The listing builds one solid part. Answer for the finished solid, in the listing's coordinates (mm). A direction names the side the tool comes from. Give positions to 0.01 mm unless a question says otherwise; leave off trailing zeros. Write each loop counter-clockwise with the first axis right and the second up, starting at its lowest first coordinate (ties: lowest second). Pieces come first, ordered by that corner, then holes. Notation, with made-up numbers: M -30,23.25 L -1,23.25 A32 cw -1,59.25 Z; hole C -38,-2.5 d4. An arc over 180 degrees is marked long. Return JSON: item names as keys, results as strings.
from build123d import *

# Parameters (mm, degrees)
F0_W     = 228.6
F0_H     = 182.245
F1_DEPTH = 7.62
F2_W     = 228.6
F2_H     = 158.7754
F3_DEPTH = 6.731
F4_W     = 2.54
F4_H     = 2.54
F5_DEPTH = 228.6
F6_W     = 20.32
F6_H     = 20.32
F7_DEPTH = 76.2
F8_W     = 81.5747073555
F8_H     = 20.3200148768
F9_DEPTH = 19.05
F10_R    = 10.16


with BuildPart() as f1:
    # F0 (on Top) → F1 (new body)
    with BuildSketch(Plane.XY):
        with Locations((53.7457112223, 38.7887536495)):
            Rectangle(F0_W, F0_H)
    extrude(amount=F1_DEPTH)

    # F2 (on face) → F3 (join)
    with BuildSketch(Plane(origin=(0, 0, 0), x_dir=(1, 0, 0), z_dir=(0, 0, -1))):
        with Locations((53.7457112223, -38.7887536495)):
            Rectangle(F2_W, F2_H)
    extrude(amount=F3_DEPTH)

    # F4 (on face) → F5 (join)
    with BuildSketch(Plane.YZ.offset(168.0457112223)):
        with Locations((119.4464536495, -5.461)):
            Rectangle(F4_W, F4_H)
        with Locations((-41.8689463505, -5.461)):
            Rectangle(F4_W, F4_H)
    extrude(amount=-F5_DEPTH)

    # F6 (on face) → F7 (join)
    with BuildSketch(Plane.XY.offset(7.62)):
        with Locations((0, 38.7887536495)):
            Rectangle(F6_W, F6_H)
        Polygon((101.8946701026, 48.9487536495), (91.7346701026, 48.9487536495), (91.7346701026, 28.6287536495), (112.0546701026, 28.6287536495), (112.0546701026, 48.9487536495), align=None)
    extrude(amount=F7_DEPTH)

    # F8 (on face) → F9 (join)
    with BuildSketch(Plane.XY.offset(83.82)):
        with Locations((50.9473536777, 38.7887610879)):
            Rectangle(F8_W, F8_H)
    extrude(amount=-F9_DEPTH)

    # F10
    f10_edges = [f1.edges().sort_by_distance(p)[0] for p in [
        (-10.16, 38.788754, 83.82),
        (112.05467, 38.788754, 83.82),
        (10.16, 38.788754, 64.77),
        (91.73467, 38.788754, 64.77),
    ]]
    fillet(f10_edges, radius=F10_R)


solid = f1.part
Item 1: Which of the six approach directions +Z, -Z, +X, -X, +Y, -Y give full straight-line access (tool end or side, diameter ignored) to faces 1 (the flat face through (-10.16, 39, 40)), 2 (the flat face through (50, 39, 64.77)), 3 (the flat face through (52, 124, 0)), 4 (the flat face through (50, 28.629, 72))?
Geometry results:
{"face 1": "+Z, -X, +Y, -Y", "face 2": "+Y, -Y", "face 3": "+X, -X, +Y", "face 4": "+Z, +X, -X, -Y"}
Item 2: A cutting plane is placed at D-D, the plane y = 75.5. Write down the section's boundary in (x, z), plus the area to 3 significant figures.
Geometry results:
{"outline": "M -60.55,-6.73 L 168.05,-6.73 L 168.05,7.62 L -60.55,7.62 Z", "area": "3,280 mm2"}
Item 3: A cutting plane is placed at A-A, the plane x = 62. Write down the section's boundary in (y, z).
Geometry results:
{"outline": "M -52.33,0 L -40.6,0 L -40.6,-4.19 L -43.14,-4.19 L -43.14,-6.73 L 120.72,-6.73 L 120.72,-4.19 L 118.18,-4.19 L 118.18,0 L 129.91,0 L 129.91,7.62 L -52.33,7.62 Z; M 28.63,64.77 L 48.95,64.77 L 48.95,83.82 L 28.63,83.82 Z"}
Item 4: A cutting plane is placed at C-C, the plane x = -45. Write down the section's boundary in (y, z), plus the area to 3 significant figures.
Geometry results:
{"outline": "M -52.33,0 L -40.6,0 L -40.6,-4.19 L -43.14,-4.19 L -43.14,-6.73 L 120.72,-6.73 L 120.72,-4.19 L 118.18,-4.19 L 118.18,0 L 129.91,0 L 129.91,7.62 L -52.33,7.62 Z", "area": "2,470 mm2"}
Item 5: Determine the mould class of faces 5 (the cylindrical face through (88.68, 38.65, 61.87)), 6 (the flat face through (52, -46, 0)), 7 (the flat face through (112.055, 39, 40)) for opening direction X: +X half, -X half, draft (parallel to the pull), parting line (faces both ways), or undercut.
Geometry results:
{"face 5": "undercut", "face 6": "draft", "face 7": "+X half"}
Item 6: A cutting plane is placed at B-B, the plane y = 35.5. Write down the section's boundary in (x, z).
Geometry results:
{"outline": "M -60.55,-6.73 L 168.05,-6.73 L 168.05,7.62 L 112.05,7.62 L 112.05,73.66 A10.16 ccw 101.89,83.82 L 0,83.82 A10.16 ccw -10.16,73.66 L -10.16,7.62 L -60.55,7.62 Z; hole M 10.16,7.62 L 91.73,7.62 L 91.73,54.61 A10.16 ccw 81.57,64.77 L 20.32,64.77 A10.16 ccw 10.16,54.61 Z"}
Item 7: Find the intervals of material crossed by line 1 (Z direction, x = 16.5, y = 120.5); line 2 (Y direction, x = 87, z = 78.5); line 3 (Z direction, x = 149.5, y = 76), in increasing order.
Geometry results:
{"line 1": "z = -6.73 to -4.19, 0 to 7.62", "line 2": "y = 28.63 to 48.95", "line 3": "z = -6.73 to 7.62"}
Item 8: Given pin 1 Ø23 at (x, z) = (26, 51.5) entering from -Y; pin 2 Ø1.3 at (x, z) = (109, -5.5) entering from -Y; pin 3 Ø6 at (x, y) = (79, -48.5) entering from -Z; pin 4 Ø3 at (x, y) = (110, 91.5) entering from +Z, each flat-ended and moving along its own axis, determine where each tip first touches the part or whether it passes through.
Geometry results:
{"pin 1": "passes through", "pin 2": "stops at y = -43.14", "pin 3": "stops at z = 0", "pin 4": "stops at z = 7.62"}
